Can you work these out from the drawing? Everything is in mm from the part's minimum corner. A direction names the side the tool comes from. Give positions to 0.01 mm unless a question says otherwise; leave off trailing zeros. Loops run counter-clockwise (first coordinate to the right, second up) from the corner with the lowest first, then second, coordinate; pieces in that order, holes last.
Q1. Will these pins go through, and if not, where does the flat tip stop? P1, Ø7.5, axis at x = 25.5, z = 17.5, coming from the +Y side; P2, Ø1.6, axis at x = 53.5, y = 7.5, coming from the -Z side; P3, Ø4, axis at x = 11.5, z = 3, coming from the +Y side; P4, Ø1.5, axis at x = 61, y = 3, coming from the +Z side.
Q2. If we section it at D-D (x = 10.5): Please give me the cut outline in (y, z).
Q3. If we section it at A-A (y = 19.75): Please give me the cut outline in (x, z), plus the area to 3 significant figures.
Q4. For the marked faces 1 and 2, which set-ups out of +Z, -Z, +X, -X, +Y, -Y let a thin tool reach every point of the face, with its end or its side?
Q5. I need wall thicknesses on line 1 (X direction, y = 0.45, z = 10); line 2 (Z direction, x = 15, y = 0.65); line 3 (Y direction, x = 53.5, z = 0.4). Which ranges of each line are inside material? Lowest first, please.
Q6. If we section it at C-C (y = 7.5): Please give me the cut outline in (x, z).
Q7. If we section it at B-B (x = 53.5): Please give me the cut outline in (y, z).
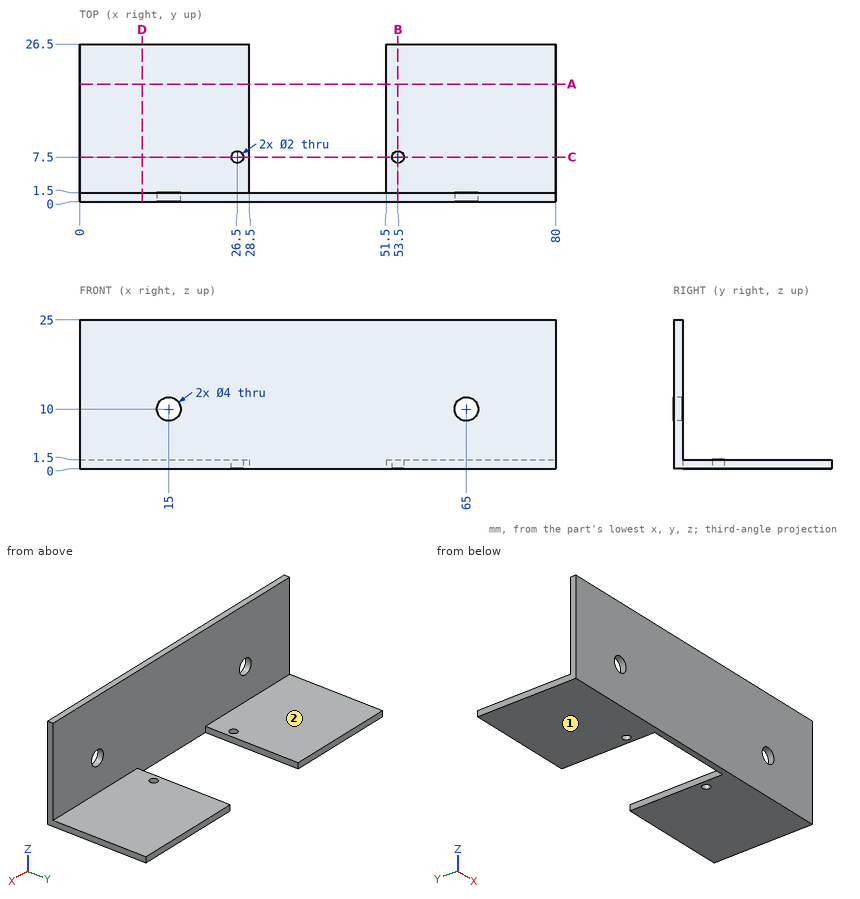
Check sheet entries:
1. P1: stops at y = 1.5
1. P2: passes through
1. P3: stops at y = 26.5
1. P4: stops at z = 1.5
2. outline: (0, 0) - (26.5, 0) - (26.5, 1.5) - (1.5, 1.5) - (1.5, 25) - (0, 25) - close
3. outline: (0, 0) - (28.5, 0) - (28.5, 1.5) - (0, 1.5) - close; (51.5, 0) - (80, 0) - (80, 1.5) - (51.5, 1.5) - close
3. area: 85.5 mm2
4. face 1: -Z, +X, -X, +Y, -Y
4. face 2: +Z, +X, -X, +Y
5. line 1: x = 0 to 13, 17 to 63, 67 to 80
5. line 2: z = 0 to 8, 12 to 25
5. line 3: y = 0 to 6.5, 8.5 to 26.5
6. outline: (0, 0) - (25.5, 0) - (25.5, 1.5) - (0, 1.5) - close; (27.5, 0) - (28.5, 0) - (28.5, 1.5) - (27.5, 1.5) - close; (51.5, 0) - (52.5, 0) - (52.5, 1.5) - (51.5, 1.5) - close; (54.5, 0) - (80, 0) - (80, 1.5) - (54.5, 1.5) - close
7. outline: (0, 0) - (6.5, 0) - (6.5, 1.5) - (1.5, 1.5) - (1.5, 25) - (0, 25) - close; (8.5, 0) - (26.5, 0) - (26.5, 1.5) - (8.5, 1.5) - close
